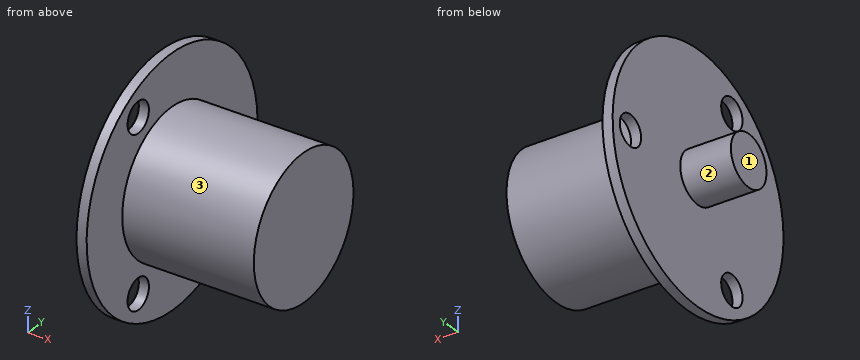
from build123d import *

# Parameters (mm, degrees)
SKETCH1_R           = 12
BOSS_EXTRUDE1_DEPTH = 1
SKETCH2_R           = 7
BOSS_EXTRUDE2_DEPTH = 13
SKETCH3_R           = 1.5
CUT_EXTRUDE1_DEPTH  = 1
SKETCH4_R           = 2.5
BOSS_EXTRUDE3_DEPTH = 5


with BuildPart() as part:
    # Sketch1 → Boss-Extrude1 (new body)
    with BuildSketch(Plane(origin=(0, 0, 0), x_dir=(0, 0, -1), z_dir=(1, 0, 0))):
        Circle(SKETCH1_R)
    extrude(amount=BOSS_EXTRUDE1_DEPTH)

    # Sketch2 → Boss-Extrude2 (add)
    with BuildSketch(Plane(origin=(1, 0, 0), x_dir=(0, 0, -1), z_dir=(1, 0, 0))):
        with Locations(Location((0, 0, 0), (0, 0, 180))):
            Circle(SKETCH2_R)
    extrude(amount=BOSS_EXTRUDE2_DEPTH)

    # Sketch3 → Cut-Extrude1 (cut)
    with BuildSketch(Plane(origin=(1, 0, 0), x_dir=(0, 0, -1), z_dir=(1, 0, 0))):
        with Locations((0, 9.5)):
            Circle(SKETCH3_R)
        with Locations((8.227241336, -4.75)):
            Circle(SKETCH3_R)
        with Locations((-8.227241336, -4.75)):
            Circle(SKETCH3_R)
    extrude(amount=-CUT_EXTRUDE1_DEPTH, mode=Mode.SUBTRACT)

    # Sketch4 → Boss-Extrude3 (add)
    with BuildSketch(Plane.ZY):
        with Locations(Location((0, 0, 0), (0, 0, 180))):
            Circle(SKETCH4_R)
    extrude(amount=BOSS_EXTRUDE3_DEPTH)


solid = part.part
Can you work these out from the model? Positions are in its coordinate system, mm. Face numbers are marked on the shaded views. A direction names the side the tool comes from. Round coordinates to 2 decimals unless told otherwise and drop trailing zeros. Order: outer loops, then holes, each group sorted by start corner. A loop starts at its lowest first (then second) coordinate and runs counter-clockwise, first axis right, second up. Notation, with made-up numbers: (10.25, 57) - (65.25, 57) arc R11 cw to (65.25, 78) - close; hole circle Ø7 at (78, 48.5). An arc over 180 degrees is marked (long way). Answer in a Markdown table with one row per item.
(1) Which directions (+Z, -Z, +X, -X, +Y, -Y) give clear straight access to the entire face, cutting with the end or side of a thin tool? Please do the marked faces 1, 2 and 3.
From the geometry:
| item | result |
|---|---|
| face 1 | +Z, -Z, -X, +Y, -Y |
| face 2 | -X |
| face 3 | +X |
(2) Suppose I cut it at C-C, the plane y = 0. Please give me the cut outline in (x, z), plus the area to 3 significant figures.
From the geometry:
| item | result |
|---|---|
| outline | (-5, -2.5) - (0, -2.5) - (0, -12) - (1, -12) - (1, -7) - (14, -7) - (14, 7) - (1, 7) - (1, 12) - (0, 12) - (0, 2.5) - (-5, 2.5) - close |
| area | 231 mm2 |
(3) For P1, Ø2.5, axis at y = -4.75, z = -8.23, coming from the -X side; P2, Ø1.5, axis at y = -4, z = 1.5, coming from the -X side; P3, Ø10, axis at x = 8, y = -9, coming from the +Z side; P4, Ø3, axis at x = 8, y = -7.5, coming from the +Z side, each with a flat end and sliding along its axis, tell me the tip position at first contact or that it passes through.
From the geometry:
| item | result |
|---|---|
| P1 | passes through |
| P2 | stops at x = 0 |
| P3 | stops at z = 5.74 |
| P4 | stops at z = 3.61 |
(4) Suppose I cut it at A-A, the plane z = 0. Please give me the cut outline in (x, y).
From the geometry:
| item | result |
|---|---|
| outline | (-5, -2.5) - (0, -2.5) - (0, -12) - (1, -12) - (1, -7) - (14, -7) - (14, 7) - (1, 7) - (1, 8) - (0, 8) - (0, 2.5) - (-5, 2.5) - close; (0, 11) - (1, 11) - (1, 12) - (0, 12) - close |
(5) Suppose I cut it at D-D, the plane x = 9.5. Please give me the cut outline in (y, z).
From the geometry:
| item | result |
|---|---|
| outline | circle Ø14 at (0, 0) |
(6) Please list where these lines run through material, in increasing order: L1, parallel to Y at x = 0.75, z = 0; L2, parallel to X at y = 1.5, z = -2.75; L3, parallel to X at y = -7, z = -3. Write a range as from..to.
From the geometry:
| item | result |
|---|---|
| L1 | y = -12..8, 11..12 |
| L2 | x = 0..14 |
| L3 | x = 0..1 |
(7) Suppose I cut it at B-B, the plane y = 8.5. Please give me the cut outline in (x, z).
From the geometry:
| item | result |
|---|---|
| outline | (0, -8.47) - (1, -8.47) - (1, -1.12) - (0, -1.12) - close; (0, 1.12) - (1, 1.12) - (1, 8.47) - (0, 8.47) - close |
